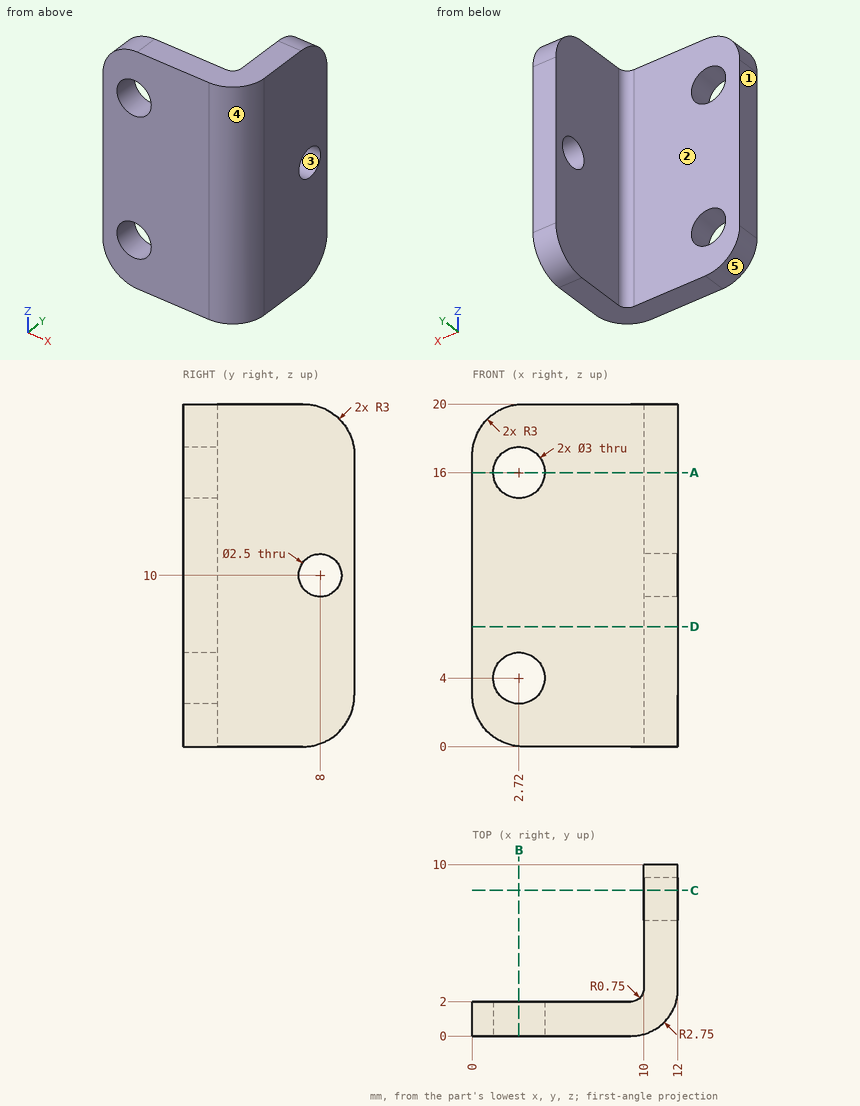
The figure shows three views and two pictorial views of one solid part (mm, origin at its lowest corner). Answer the questions. A direction names the side the tool comes from. Coordinates: 2 decimals unless noted, no trailing zeros. Loops run counter-clockwise (first coordinate to the right, second up) from the corner with the lowest first, then second, coordinate; pieces in that order, holes last. Notation, with made-up numbers: (-38, 31.25) - (-11, 31.25) arc R17 ccw to (-11, 56.25) - close; hole circle Ø6 at (-3.5, 4.25). An arc over 180 degrees is marked (long way). Answer in a Markdown table with one row per item.
Q1. Find section D-D on z = 7. Write down the section's boundary in (x, y), plus the area to 3 significant figures.
Here are the results:
| item | result |
|---|---|
| outline | (0, 0) - (9.25, 0) arc R2.75 ccw to (12, 2.75) - (12, 10) - (10, 10) - (10, 2.75) arc R0.75 cw to (9.25, 2) - (0, 2) - close |
| area | 38.5 mm^2 |
Q2. Find section A-A on z = 16. Write down the section's boundary in (x, y), plus the area to 3 significant figures.
Here are the results:
| item | result |
|---|---|
| outline | (0, 0) - (1.22, 0) - (1.22, 2) - (0, 2) - close; (4.22, 0) - (9.25, 0) arc R2.75 ccw to (12, 2.75) - (12, 10) - (10, 10) - (10, 2.75) arc R0.75 cw to (9.25, 2) - (4.22, 2) - close |
| area | 32.5 mm^2 |
Q3. Find section B-B on x = 2.72. Write down the section's boundary in (y, z), plus the area to 3 significant figures.
Here are the results:
| item | result |
|---|---|
| outline | (0, 0.01) - (2, 0.01) - (2, 2.5) - (0, 2.5) - close; (0, 5.5) - (2, 5.5) - (2, 14.5) - (0, 14.5) - close; (0, 17.5) - (2, 17.5) - (2, 19.99) - (0, 19.99) - close |
| area | 27.9 mm^2 |
Q4. Given P1, Ø4, axis at x = 2.72, z = 4, coming from the +Y side; P2, Ø2, axis at y = 7, z = 14, coming from the -X side, each flat-ended and moving along its own axis, determine where each tip first touches the part or whether it passes through.
Here are the results:
| item | result |
|---|---|
| P1 | stops at y = 2 |
| P2 | stops at x = 10 |
Q5. Find section C-C on y = 8.5. Write down the section's boundary in (x, z), plus the area to 3 significant figures.
Here are the results:
| item | result |
|---|---|
| outline | (10, 0.4) - (12, 0.4) - (12, 8.85) - (10, 8.85) - close; (10, 11.15) - (12, 11.15) - (12, 19.6) - (10, 19.6) - close |
| area | 33.8 mm^2 |
Q6. Straight lines are drawn through the part: line 1 along Y through (x, z) = (6.75, 12.5); line 2 along X through (y, z) = (5.75, 15); line 3 along Z through (x, y) = (10.8, 8). For each, find the intervals that lie inside material, in ascending order. Write a range as [from, to].
Here are the results:
| item | result |
|---|---|
| line 1 | y = [0, 2] |
| line 2 | x = [10, 12] |
| line 3 | z = [0.17, 8.75], [11.25, 19.83] |
Q7. For the marked faces 1 and 2, determine the directions among +Z, -Z, +X, -X, +Y, -Y from which every point of the face is accessible in a straight line to the end or side of a thin tool.
Here are the results:
| item | result |
|---|---|
| face 1 | +Z, -Z, -X, +Y, -Y |
| face 2 | +Z, -Z, -X, +Y |
Q8. The mould has two halves that part along Z. Classify the marked faces 3, 4 and 5: pulls with the +Z half, pulls with the -Z half, needs draft (parallel to the pull), parting line crosses it, or undercut.
Here are the results:
| item | result |
|---|---|
| face 3 | undercut |
| face 4 | needs draft |
| face 5 | pulls with the -Z half |
